Here's how the part is built. I have some questions about the finished solid (model axes, mm). A direction names the side the tool comes from. Round coordinates to 2 decimals unless told otherwise and drop trailing zeros. Loops run counter-clockwise (first coordinate to the right, second up) from the corner with the lowest first, then second, coordinate; pieces in that order, holes last. Notation, with made-up numbers: M 81,-21 L 130,-21 A21 cw 130,13 Z; hole C -6,-38 d11. An arc over 180 degrees is marked long. Answer as a JSON object with one key per item and string values.
from build123d import *

# Parameters (mm, degrees)
SKIZZE1_R                            = 2.1
AUFSATZ_LINEAR_AUSTRAGEN1_DEPTH      = 10
SKIZZE2_R                            = 1.5
SCHNITT_LINEAR_AUSTRAGEN1_DEPTH      = 8
SCHNITT_LINEAR_AUSTRAGEN3_DEPTH      = 2.8
SCHNITT_LINEAR_AUSTRAGEN5_DEPTH      = 69.862823313
SCHNITT_LINEAR_AUSTRAGEN5_DEPTH_BACK = 69.862823313
SKIZZE7_R                            = 10
FASE1_SIZE                           = 3
SCHNITT_LINEAR_AUSTRAGEN4_DEPTH      = 10
VERRUNDUNG1_R                        = 2
FASE2_SIZE                           = 1
FASE3_SIZE                           = 2.5
SKIZZE8_R                            = 3.6
SCHNITT_LINEAR_AUSTRAGEN6_DEPTH      = 3


with BuildPart() as part:
    # Skizze1 → Aufsatz-Linear austragen1 (new body)
    with BuildSketch(Plane.XY):
        Polygon((28.287001282, 57.370618027), (28.287001282, 0), (-13.088781156, 0), (-13.088781156, 27.348243657), (-13.088781156, 53.715647777), (-13.088781156, 57.370618027), (-13.088781156, 62.370618027), (28.287001282, 62.370618027), align=None)
        with Locations((-8.088781156, 23.031945717)):
            Circle(SKIZZE1_R, mode=Mode.SUBTRACT)
        with Locations(Location((-8.088781156, 58.031945717, 0), (0, 0, 180))):
            Circle(SKIZZE1_R, mode=Mode.SUBTRACT)
    extrude(amount=AUFSATZ_LINEAR_AUSTRAGEN1_DEPTH)

    # Skizze2 → Schnitt-Linear austragen1 (cut)
    with BuildSketch(Plane.XZ):
        with Locations((-7, 5)):
            Circle(SKIZZE2_R)
        with Locations((6.18, 5)):
            Circle(SKIZZE2_R)
        with Locations((19.36, 5)):
            Circle(SKIZZE2_R)
    extrude(amount=-SCHNITT_LINEAR_AUSTRAGEN1_DEPTH, mode=Mode.SUBTRACT)

    # Skizze4 → Schnitt-Linear austragen3 (cut)
    with BuildSketch(Plane.XY.offset(10)):
        Polygon((-15.095168359, 10), (28.287001282, 10), (36.093332102, 46.989971623), (30.429094825, 65.957451721), (-16.081030445, 65.957451721), (-16.081030445, 27.753515123), align=None)
    extrude(amount=-SCHNITT_LINEAR_AUSTRAGEN3_DEPTH, mode=Mode.SUBTRACT)

    # Skizze7 → Schnitt-Linear austragen5 (cut, two sides: drawn at the far end of the back side and taken through both)
    with BuildSketch(Plane.XY.offset(7.2).offset(-SCHNITT_LINEAR_AUSTRAGEN5_DEPTH_BACK)):
        with Locations((-0.088781156, 40.531945717)):
            Circle(SKIZZE7_R)
    extrude(amount=SCHNITT_LINEAR_AUSTRAGEN5_DEPTH + SCHNITT_LINEAR_AUSTRAGEN5_DEPTH_BACK, mode=Mode.SUBTRACT)

    # Fase1
    # the kernel refuses this chamfer: 3 mm, written as the material it takes off along each edge
    with BuildSketch(Plane(origin=(-20.80383012, 10, 10), x_dir=(0, -0.9996219169112969, 0.027495876610586202), z_dir=(1, 0, 0))) as fase1_piece_1_section:
        Polygon((FASE1_SIZE * 0.999621916911, FASE1_SIZE * 0.0274958766106), (-FASE1_SIZE * 0.0274958766106, FASE1_SIZE * 0.999621916911), (0, 0), align=None)
    fase1_piece_1 = extrude(amount=56.805880365, mode=Mode.PRIVATE)
    fase1_piece_1 = split(fase1_piece_1, bisect_by=Plane(origin=(7.599110063, 8.999392985, 7.2), z_dir=(0, 0, 1)), keep=Keep.TOP, mode=Mode.PRIVATE)
    add(fase1_piece_1, mode=Mode.SUBTRACT)

    # Skizze5 → Schnitt-Linear austragen4 (cut)
    with BuildSketch(Plane(origin=(0, 0, 0), x_dir=(-1, 0, 0), z_dir=(0, 0, -1))):
        Polygon((-24.81273389, 11.736777957), (-9.824335871, 62.370618027), (-28.287001282, 62.370618027), (-28.287001282, 0), (-24.81273389, 0), align=None)
    extrude(amount=-SCHNITT_LINEAR_AUSTRAGEN4_DEPTH, mode=Mode.SUBTRACT)

    # Verrundung1
    verrundung1_edges = [part.edges().sort_by_distance(p)[0] for p in [
        (9.824335871, 62.370618027, 3.6),
        (-13.088781156, 62.370618027, 3.6),
    ]]
    fillet(verrundung1_edges, radius=VERRUNDUNG1_R)

    # Fase2
    fase2_edges = [part.edges().sort_by_distance(p)[0] for p in [
        (24.81273389, 10.768388979, 7.2),
        (24.81273389, 3.5, 10),
        (-13.088781156, 35.085309014, 7.2),
        (-1.379099888, 62.370618027, 7.2),
        (17.530529072, 36.337538735, 7.2),
        (9.527376482, 61.973016693, 7.2),
        (-12.502994718, 61.78483159, 7.2),
        (-10.088781156, 40.531945717, 7.2),
        (-13.088781156, 8.4, 8.6),
        (24.81273389, 8.4, 8.6),
    ]]
    chamfer(fase2_edges, length=FASE2_SIZE)

    # Fase3
    fase3_edges = [part.edges().sort_by_distance(p)[0] for p in [
        (-13.088781156, 2.792893219, 10),
    ]]
    chamfer(fase3_edges, length=FASE3_SIZE)

    # Skizze8 → Schnitt-Linear austragen6 (cut)
    with BuildSketch(Plane(origin=(0, 0, 0), x_dir=(-1, 0, 0), z_dir=(0, 0, -1))):
        with Locations((8.088781156, 23.031945717)):
            Circle(SKIZZE8_R)
    extrude(amount=-SCHNITT_LINEAR_AUSTRAGEN6_DEPTH, mode=Mode.SUBTRACT)


solid = part.part
Item 1: I want a section at D-D on x = -7. Count the separate pieces of the cut face and the enclosed holes in it, plus the area to 3 significant figures.
Solution:
{"separate pieces": "4", "enclosed holes": "0", "area": "281 mm2"}
Item 2: I want a section at C-C on y = 27.5. List the corners of the cut face in (x, z) for me, plus the area to 3 significant figures.
Solution:
{"outline": "M -13.09,0 L 20.15,0 L 20.15,6.2 L 19.1,7.2 L -12.09,7.2 L -13.09,6.2 Z", "area": "238 mm2"}
Item 3: I want a section at A-A on z = 1. List the corners of the cut face in (x, y) for me.
Solution:
{"outline": "M -13.09,0 L 24.81,0 L 24.81,11.74 L 10.25,60.94 A2 ccw 8.33,62.37 L -11.09,62.37 A2 ccw -13.09,60.37 Z; hole C -8.09,23.03 d7.2; hole C -8.09,58.03 d4.2; hole C -0.09,40.53 d20"}
Item 4: We'd pull the mould along Y, two halves only. Please class faces 1 (the face through (20.79, 3.94, 5.45)), 2 (the face through (17.146, 35.849, 6.707)), 3 (the face through (-7.308, 19.518, 1.479)): +Y half, -Y half, draft (parallel to the pull), parting line (faces both ways), or undercut.
Solution:
{"face 1": "draft", "face 2": "+Y half", "face 3": "undercut"}
Item 5: I want a section at B-B on x = 12. List the corners of the cut face in (y, z) for me, plus the area to 3 significant figures.
Solution:
{"outline": "M 0,0 L 55.02,0 L 55.02,6.2 L 51.5,7.2 L 9.8,7.2 L 7,10 L 0,10 Z", "area": "418 mm2"}
Item 6: For faces 4 (the face through (6, 30, 7.2)), 5 (the face through (19, 8, 5)), 6 (the face through (-10, 21, 3)), which set-ups out of +Z, -Z, +X, -X, +Y, -Y let a thin tool reach every point of the face, with its end or its side?
Solution:
{"face 4": "+Z, +X, -X, +Y", "face 5": "-Y", "face 6": "-Z"}
Item 7: For P1, Ø4.5, axis at x = -8.09, y = 23.03, coming from the -Z side; P2, Ø3, axis at x = 1, y = 47, coming from the -Z side; P3, Ø4, axis at x = 20.5, y = 19, coming from the +Z side; P4, Ø1.5, axis at x = -3.5, z = 7, coming from the +Y side, each with a flat end and sliding along its axis, tell me the tip position at first contact or that it passes through.
Solution:
{"P1": "stops at z = 3", "P2": "passes through", "P3": "stops at z = 7.2", "P4": "stops at y = 62.32"}
Item 8: If I drill on L1, parallel to Z at x = 12, y = 44; L2, parallel to Z at x = 6, y = 4; L3, parallel to X at y = 35, z = 1.25, over which ranges is the centre line in solid material (lowest first)? Write a range as from..to.
Solution:
{"L1": "z = 0..7.2", "L2": "z = 0..3.51, 6.49..10", "L3": "x = -13.09..-8.42, 8.24..17.93"}
